from build123d import *

# Parameters (mm, degrees)
SKETCH1_W               = 30.1
SKETCH1_H               = 16
EXTRUDE1_DEPTH          = 7.2
SKETCH6_R               = 0.498915
CUT_EXTRUDE1_DEPTH      = 0.1
CUT_EXTRUDE2_DEPTH      = 1
CUT_EXTRUDE2_DEPTH_BACK = 31.1
CUT_EXTRUDE3_DEPTH      = 1
CUT_EXTRUDE3_DEPTH_BACK = 17
LPATTERN1_COUNT         = 2
LPATTERN1_PITCH         = 9.06
LPATTERN2_COUNT         = 2
LPATTERN2_PITCH         = 9.06
BOSS_EXTRUDE4_START     = -1
SKETCH11_R              = 0.225
BOSS_EXTRUDE4_DEPTH     = 2.8
LPATTERN3_COUNT         = 6
LPATTERN3_PITCH         = 2.54
LPATTERN3_COUNT_DIR2    = 2
LPATTERN3_PITCH_DIR2    = 12.7


with BuildPart() as part:
    # Sketch1 → Extrude1 (new body)
    with BuildSketch(Plane(origin=(0, 0, 0), x_dir=(1, 0, 0), z_dir=(0, 1, 0))):
        Rectangle(SKETCH1_W, SKETCH1_H)
    extrude(amount=-EXTRUDE1_DEPTH)

    # Sketch6 → Cut-Extrude1 (cut)
    with BuildSketch(Plane(origin=(0, 0, 0), x_dir=(-1, 0, 0), z_dir=(0, 1, 0))):
        with Locations((-3.136417605, 4.601105)):
            Circle(SKETCH6_R)
        Polygon((1.899392179, -5.031807345), (1.818099503, -5.10002), (-2.815721224, -5.10002), (-2.872958438, -5.031807345), (-1.993362607, -4.293738808), (1.280079142, -4.293738808), align=None)
        Polygon((-2.771014452, -0.541251787), (-3.136417605, -4.717828937), (-3.051123094, -4.819478977), (-2.191884627, -4.098492296), (-1.893012763, -0.682371264), (-2.325269688, -0.16722752), align=None)
        Polygon((1.729773181, 0.44348), (-1.804005322, 0.44348), (-2.240747865, 0.077009494), (-1.804005322, -0.44348), (1.729773181, -0.44348), (2.166515723, -0.077009494), align=None)
        Polygon((1.379758426, -3.981324201), (1.658740499, -0.792544509), (2.198389312, -0.33972539), (2.551851384, -0.760965084), (2.200290566, -4.77932362), (2.111720548, -4.85364269), align=None)
        Polygon((-1.276746018, 4.21306), (-2.008340937, 5.011455754), (-1.919776691, 5.10002), (2.680970165, 5.10002), (2.766330848, 5.014659317), (1.8915387, 4.21306), align=None)
        Polygon((-1.481100864, 4.025803284), (-2.204519978, 4.815276713), (-2.311761335, 4.708035356), (-2.66642341, 0.654229291), (-2.348850987, 0.275761216), (-1.766430556, 0.764469985), align=None)
        Polygon((2.078795416, 4.008705154), (2.962509889, 4.818480275), (3.033756345, 4.74723382), (2.674290947, 0.638525521), (2.193846693, 0.235384926), (1.790706097, 0.715829179), align=None)
    cut_extrude1 = extrude(amount=-CUT_EXTRUDE1_DEPTH, mode=Mode.SUBTRACT)

    # Sketch12 → Cut-Extrude2 (cut, two sides)
    with BuildSketch(Plane.ZY.offset(15.05)) as cut_extrude2_sk:
        Polygon((-22.464786823, -46.104536903), (-6.35, -7.2), (-5.935786438, -6.2), (5.935786438, -6.2), (6.35, -7.2), (22.464786823, -46.104536903), (22.464786823, -130.324471503), (-22.464786823, -130.324471503), align=None)
    extrude(amount=CUT_EXTRUDE2_DEPTH, mode=Mode.SUBTRACT)
    extrude(cut_extrude2_sk.sketch, amount=-CUT_EXTRUDE2_DEPTH_BACK, mode=Mode.SUBTRACT)

    # Sketch13 → Cut-Extrude3 (cut, two sides)
    with BuildSketch(Plane(origin=(0, 0, -8), x_dir=(-1, 0, 0), z_dir=(0, 0, -1))) as cut_extrude3_sk:
        Polygon((-42.431282579, -69.457786403), (-13.4, -7.2), (-12.933692342, -6.2), (12.933692342, -6.2), (13.4, -7.2), (42.431282579, -69.457786403), (42.431282579, -206.845520004), (-42.431282579, -206.845520004), align=None)
    extrude(amount=CUT_EXTRUDE3_DEPTH, mode=Mode.SUBTRACT)
    extrude(cut_extrude3_sk.sketch, amount=-CUT_EXTRUDE3_DEPTH_BACK, mode=Mode.SUBTRACT)

    # LPattern1: Cut-Extrude1 ×2
    with Locations(*[(i * LPATTERN1_PITCH, 0, 0) for i in range(1, LPATTERN1_COUNT)]):
        add(cut_extrude1, mode=Mode.SUBTRACT)

    # LPattern2: Cut-Extrude1 ×2
    with Locations(*[(-i * LPATTERN2_PITCH, 0, 0) for i in range(1, LPATTERN2_COUNT)]):
        add(cut_extrude1, mode=Mode.SUBTRACT)

    # Sketch11 → Boss-Extrude4 (add)
    with BuildSketch(Plane.XZ.offset(7.2).offset(BOSS_EXTRUDE4_START)):
        with Locations((6.35, 6.35)):
            Circle(SKETCH11_R)
    boss_extrude4 = extrude(amount=BOSS_EXTRUDE4_DEPTH)

    # LPattern3: Boss-Extrude4 6 × 2
    with Locations(*[(-i * LPATTERN3_PITCH, 0, -j * LPATTERN3_PITCH_DIR2) for i in range(LPATTERN3_COUNT) for j in range(LPATTERN3_COUNT_DIR2) if (i, j) != (0, 0)]):
        add(boss_extrude4)


solid = part.part
Verification items for the finished model (mm, model axes). A direction names the side the tool comes from. Coordinates: 2 decimals unless noted, no trailing zeros. Write each loop counter-clockwise with the first axis right and the second up, starting at its lowest first coordinate (ties: lowest second). Pieces come first, ordered by that corner, then holes. Notation, with made-up numbers: (-2, 86) - (13, 86) arc R30 ccw to (13, 112) - close; hole circle Ø3 at (36.25, -21). An arc over 180 degrees is marked (long way). Answer as a JSON object with one key per item and string values.
(1) Cross-section at A-A on y = -6.5. Give the number of separate pieces and of enclosed holes in the cut face, plus the area to 3 significant figures.
Report:
{"separate pieces": "16", "enclosed holes": "0", "area": "17.2 mm^2"}
(2) Tool access check on faces 3 (the flat face through (-14.01, -6.69, 6.14)), 4 (the flat face through (13.17, -6.71, -6.98)), 5 (the flat face through (-11, -0.1, -3)), 6 (the flat face through (0, -6.2, 0)). Record the directions out of +Z, -Z, +X, -X, +Y, -Y that give a thin tool (end or side, any length) a straight path to the whole face; none if there is none.
Report:
{"face 3": "-X, -Y", "face 4": "+Z, -Z, -Y", "face 5": "+Y", "face 6": "-Y"}
(3) Cross-section at C-C on z = -1.75. Record the cut outline in (x, y), plus the area to 3 significant figures.
Report:
{"outline": "(-15.05, -6.2) - (15.05, -6.2) - (15.05, 0) - (11.94, 0) - (11.94, -0.1) - (11.05, -0.1) - (11.05, 0) - (7.49, 0) - (7.49, -0.1) - (6.59, -0.1) - (6.59, 0) - (2.88, 0) - (2.88, -0.1) - (1.99, -0.1) - (1.99, 0) - (-1.57, 0) - (-1.57, -0.1) - (-2.47, -0.1) - (-2.47, 0) - (-6.18, 0) - (-6.18, -0.1) - (-7.07, -0.1) - (-7.07, 0) - (-10.63, 0) - (-10.63, -0.1) - (-11.53, -0.1) - (-11.53, 0) - (-15.05, 0) - close", "area": "186 mm^2"}
(4) Thickness scan on line 1 along X through (y, z) = (-7.5, -6.5); line 2 along Y through (x, z) = (12, -5.75); line 3 along Y through (x, z) = (7, -0.5). Record the ranges inside material, lowest first.
Report:
{"line 1": "-6.52 to -6.18, -3.98 to -3.64, -1.44 to -1.1, 1.1 to 1.44, 3.64 to 3.98, 6.18 to 6.52", "line 2": "-6.2 to 0", "line 3": "-6.2 to -0.1"}
(5) Cross-section at D-D on z = -5.5. Record the cut outline in (x, y), plus the area to 3 significant figures.
Report:
{"outline": "(-15.05, -6.2) - (15.05, -6.2) - (15.05, 0) - (-15.05, 0) - close", "area": "187 mm^2"}
(6) Gauge pin test, flat ends, axial feed: pin 1 Ø0.5 at (x, z) = (14.5, 7) entering from -Y; pin 2 Ø5 at (x, z) = (7.5, 1) entering from -Y. Record the tip position at first contact, or that the pin passes through.
Report:
{"pin 1": "y = -7.2", "pin 2": "y = -6.2"}
(7) Mould release check, pull along Z, two halves, no side actions. Record for faces 1 (the flat face through (13.17, -6.71, 6.95)), 2 (the flat face through (-11.5, -0.1, 2.6)): pulls with the +Z half, pulls with the -Z half, needs draft (parallel to the pull), parting line crosses it, or undercut.
Report:
{"face 1": "needs draft", "face 2": "undercut"}
